from build123d import *

# Parameters (mm, degrees)
SKETCH1_W               = 20
SKETCH1_H               = 20
BOSS_EXTRUDE1_DEPTH     = 20
CUT_EXTRUDE1_DEPTH      = 31
CUT_EXTRUDE1_DEPTH_BACK = 31
SKETCH3_R               = 4
CUT_EXTRUDE2_DEPTH      = 31
SKETCH4_R               = 4
CUT_EXTRUDE3_DEPTH      = 25.494897428
SKETCH5_W               = 15
SKETCH5_H               = 15
CUT_EXTRUDE5_DEPTH      = 17.5


with BuildPart() as part:
    # Sketch1 → Boss-Extrude1 (new body)
    with BuildSketch(Plane(origin=(0, 0, 0), x_dir=(1, 0, 0), z_dir=(0, 1, 0))):
        Rectangle(SKETCH1_W, SKETCH1_H)
    extrude(amount=BOSS_EXTRUDE1_DEPTH)

    # Sketch2 → Cut-Extrude1 (cut, two sides: drawn at the far end of the back side and taken through both)
    with BuildSketch(Plane.XY.offset(10).offset(-CUT_EXTRUDE1_DEPTH_BACK)):
        Polygon((-10, 0), (10, 20), (-10, 20), align=None)
    extrude(amount=CUT_EXTRUDE1_DEPTH + CUT_EXTRUDE1_DEPTH_BACK, mode=Mode.SUBTRACT)

    # Sketch3 → Cut-Extrude2 (cut, through all)
    with BuildSketch(Plane(origin=(10, 0, 0), x_dir=(0, 0, -1), z_dir=(1, 0, 0))):
        with Locations((0, 10)):
            Circle(SKETCH3_R)
    extrude(amount=-CUT_EXTRUDE2_DEPTH, mode=Mode.SUBTRACT)

    # Sketch4 → Cut-Extrude3 (cut, through all)
    with BuildSketch(Plane.XZ):
        with Locations(Location((0, 0, 0), (0, 0, 270))):
            Circle(SKETCH4_R)
    extrude(amount=-CUT_EXTRUDE3_DEPTH, mode=Mode.SUBTRACT)

    # Sketch5 → Cut-Extrude5 (cut)
    with BuildSketch(Plane(origin=(0, 20, 0), x_dir=(1, 0, 0), z_dir=(0, 1, 0))):
        Rectangle(SKETCH5_W, SKETCH5_H)
    extrude(amount=-CUT_EXTRUDE5_DEPTH, mode=Mode.SUBTRACT)


solid = part.part
Geometry: final body of the model. Coordinates: model frame, mm. A direction names the side the tool comes from. Coordinates: 2 decimals unless noted, no trailing zeros. Order: outer loops, then holes, each group sorted by start corner. A loop starts at its lowest first (then second) coordinate and runs counter-clockwise, first axis right, second up.
(1) Section query A-A (y = 10). Return the cut outline in (x, z), plus the area to 3 significant figures.
(2) Section query D-D (x = -7). Return the cut outline in (y, z).
(3) Material intervals for probe 1 along Z at (x, y) = (2.5, 2.75); probe 2 along X at (y, z) = (11.5, -4.75); probe 3 along X at (y, z) = (1.9, 0), sorted ascending.
(4) First-contact query: pin 1 (4.5 mm diameter, centred on x = -2, y = 13, fed in from +Z); pin 2 (2 mm diameter, centred on x = 1, z = -5, fed in from +Y); pin 3 (2 mm diameter, centred on y = 6, z = 0, fed in from -X); pin 4 (8 mm diameter, centred on x = -6, z = -4, fed in from +Y). Flat tips, straight axial feed; report the tip coordinate or a pass-through.
(5) Access query for faces 5 (the face through (-3, 2.5, -3)), 6 (the face through (4, 5, 10)). Directions: +Z, -Z, +X, -X, +Y, -Y. A direction counts if a zero-diameter tool reaches every point of the face in a straight line with its end or side. Return the directions, or none.
(6) Draft query along Z for faces 1 (the face through (4, 5, -10)), 2 (the face through (4.3, 0, -0.1)), 3 (the face through (7.5, 7, 3)), 4 (the face through (-3.905, 1.232, 0.867)). Return one class per face: pulls with the +Z half, pulls with the -Z half, needs draft (parallel to the pull), parting line crosses it, or undercut.
(7) Section query B-B (z = 0). Return the cut outline in (x, y), plus the area to 3 significant figures.
(8) Section query C-C (x = 8). Return the cut outline in (y, z).
Solution:
1. outline: (0, -10) - (10, -10) - (10, -4) - (7.5, -4) - (7.5, -7.5) - (0, -7.5) - close; (0, 7.5) - (7.5, 7.5) - (7.5, 4) - (10, 4) - (10, 10) - (0, 10) - close
1. area: 67.5 mm2
2. outline: (0, -10) - (3, -10) - (3, -7.5) - (2.5, -7.5) - (2.5, 7.5) - (3, 7.5) - (3, 10) - (0, 10) - close
3. probe 1: z = -10 to -7.5, 7.5 to 10
3. probe 2: x = 7.5 to 10
3. probe 3: x = -8.1 to -4, 4 to 10
4. pin 1: passes through
4. pin 2: stops at y = 2.5
4. pin 3: stops at x = 7.5
4. pin 4: stops at y = 5.94
5. face 5: -X, +Y
5. face 6: +Z, +X, -X, +Y, -Y
6. face 1: pulls with the -Z half
6. face 2: needs draft
6. face 3: undercut
6. face 4: undercut
7. outline: (-10, 0) - (-4, 0) - (-4, 2.5) - (-7.5, 2.5) - close; (4, 0) - (10, 0) - (10, 6) - (7.5, 6) - (7.5, 2.5) - (4, 2.5) - close; (7.5, 14) - (10, 14) - (10, 20) - (7.5, 17.5) - close
7. area: 47.5 mm2
8. outline: (0, -10) - (18, -10) - (18, 10) - (0, 10) - close; hole circle Ø8 at (10, 0)
